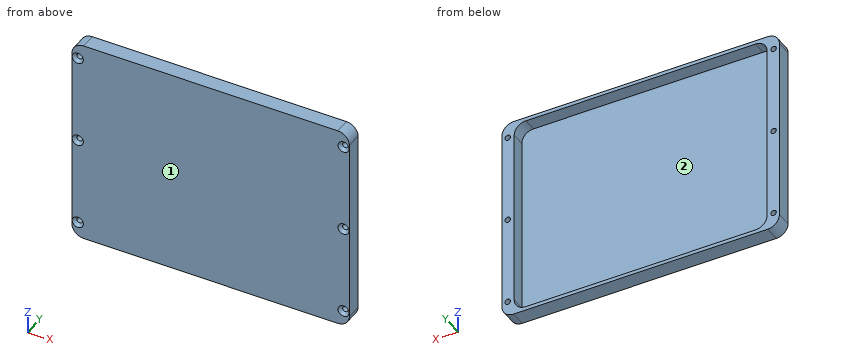
```python
from build123d import *

# Parameters (mm, degrees)
SKETCH1_W                                         = 226.949
SKETCH1_H                                         = 171.45
BOSS_EXTRUDE1_DEPTH                               = 12.7
CUT_EXTRUDE1_DEPTH                                = 11.1125
CSK_FOR_8_FLAT_HEAD_SOCKET_CAP_SCREW1_D           = 4.4958
CSK_FOR_8_FLAT_HEAD_SOCKET_CAP_SCREW1_CSINK_D     = 9.1186
CSK_FOR_8_FLAT_HEAD_SOCKET_CAP_SCREW1_CSINK_ANGLE = 82
FILLET1_R                                         = 9.525


with BuildPart() as part:
    # Sketch1 → Boss-Extrude1 (new body)
    with BuildSketch(Plane(origin=(0, 0, 0), x_dir=(1, 0, 0), z_dir=(0, 1, 0))):
        with Locations((113.4745, 85.725)):
            Rectangle(SKETCH1_W, SKETCH1_H)
    extrude(amount=BOSS_EXTRUDE1_DEPTH)

    # Sketch2 → Cut-Extrude1 (cut)
    with BuildSketch(Plane(origin=(0, 12.7, 0), x_dir=(1, 0, 0), z_dir=(0, 1, 0))):
        with BuildLine():
            Line((19.558, 2.921), (207.391, 2.921))
            ThreePointArc((207.391, 2.921), (214.126192091, 5.710807909), (216.916, 12.446))
            Line((216.916, 12.446), (216.916, 159.004))
            ThreePointArc((216.916, 159.004), (214.126192091, 165.739192091), (207.391, 168.529))
            Line((207.391, 168.529), (19.558, 168.529))
            ThreePointArc((19.558, 168.529), (12.822807909, 165.739192091), (10.033, 159.004))
            Line((10.033, 159.004), (10.033, 12.446))
            ThreePointArc((10.033, 12.446), (12.822807909, 5.710807909), (19.558, 2.921))
        make_face()
    extrude(amount=-CUT_EXTRUDE1_DEPTH, mode=Mode.SUBTRACT)

    # CSK for #8 Flat Head Socket Cap Screw1 (through all)
    with Locations(Plane.XZ):
        with Locations((4.7625, -12.7), (4.7625, -158.75), (4.7625, -85.725)):
            csk_for_8_flat_head_socket_cap_screw1 = CounterSinkHole(CSK_FOR_8_FLAT_HEAD_SOCKET_CAP_SCREW1_D / 2, CSK_FOR_8_FLAT_HEAD_SOCKET_CAP_SCREW1_CSINK_D / 2, counter_sink_angle=CSK_FOR_8_FLAT_HEAD_SOCKET_CAP_SCREW1_CSINK_ANGLE)

    # Mirror1: CSK for #8 Flat Head Socket Cap Screw1 across plane
    add(csk_for_8_flat_head_socket_cap_screw1.mirror(Plane(origin=(113.4745, 0, 0), x_dir=(0, 0, 1), z_dir=(1, 0, 0))), mode=Mode.SUBTRACT)

    # Fillet1
    fillet1_edges = [part.edges().sort_by_distance(p)[0] for p in [
        (0, 6.35, -171.45),
        (226.949, 6.35, -171.45),
        (226.949, 6.35, 0),
        (0, 6.35, 0),
    ]]
    fillet(fillet1_edges, radius=FILLET1_R)


solid = part.part
```
Model file for the job. Use its own axes, mm. Face numbers are marked on the shaded views. Coordinates: 2 decimals unless noted, no trailing zeros. Order: outer loops, then holes, each group sorted by start corner. A loop starts at its lowest first (then second) coordinate and runs counter-clockwise, first axis right, second up. Notation, with made-up numbers: M -23,-39.5 L 34,-39.5 A13 ccw 34,-25.5 Z; hole C 81.5,88 d8. An arc over 180 degrees is marked long. Answer as CSV lines item,"result".
(1) Pull direction Z, two halves, no side cores. Call the marked faces 1 and 2: +Z half, -Z half, draft (parallel to the pull), parting line (faces both ways), or undercut.
Geometry says:
face 1,"draft"
face 2,"undercut"
(2) Band-saw the part on C-C, the plane y = 9.5. State how many separate pieces and enclosed holes the cut face has, then the cut area to 3 significant figures.
Geometry says:
separate pieces,"1"
enclosed holes,"7"
area,"4,550 mm2"
(3) Wall check: line 1 along X through (y, z) = (9.25, -158.75); line 2 along X through (y, z) = (4, -105); line 3 along Z through (x, y) = (100, 11.5). Give the ranges that are in metal, low to high.
Geometry says:
line 1,"x = 0 to 2.51, 7.01 to 10.03, 216.92 to 219.94, 224.43 to 226.95"
line 2,"x = 0 to 10.03, 216.92 to 226.95"
line 3,"z = -171.45 to -168.53, -2.92 to 0"
(4) Flat gauge pins, fed straight in: pin 1 (7 mm diameter, centred on x = 4.76, z = -158.75, fed in from -Y); pin 2 (12 mm diameter, centred on x = 182, z = -44.5, fed in from +Y); pin 3 (4 mm diameter, centred on x = 222.19, z = -12.7, fed in from -Y); pin 4 (5 mm diameter, centred on x = 222.19, z = -158.75, fed in from -Y). Where does each tip first touch, or does it go through?
Geometry says:
pin 1,"stops at y = 1.22"
pin 2,"stops at y = 1.59"
pin 3,"passes through"
pin 4,"stops at y = 2.36"
(5) Band-saw the part on B-B, the plane x = 102.5. List the corners of the cut face in (y, z).
Geometry says:
outline,"M 0,-171.45 L 12.7,-171.45 L 12.7,-168.53 L 1.59,-168.53 L 1.59,-2.92 L 12.7,-2.92 L 12.7,0 L 0,0 Z"
(6) Band-saw the part on A-A, the plane z = -68.5. List the corners of the cut face in (x, y).
Geometry says:
outline,"M 0,0 L 226.95,0 L 226.95,12.7 L 216.92,12.7 L 216.92,1.59 L 10.03,1.59 L 10.03,12.7 L 0,12.7 Z"
